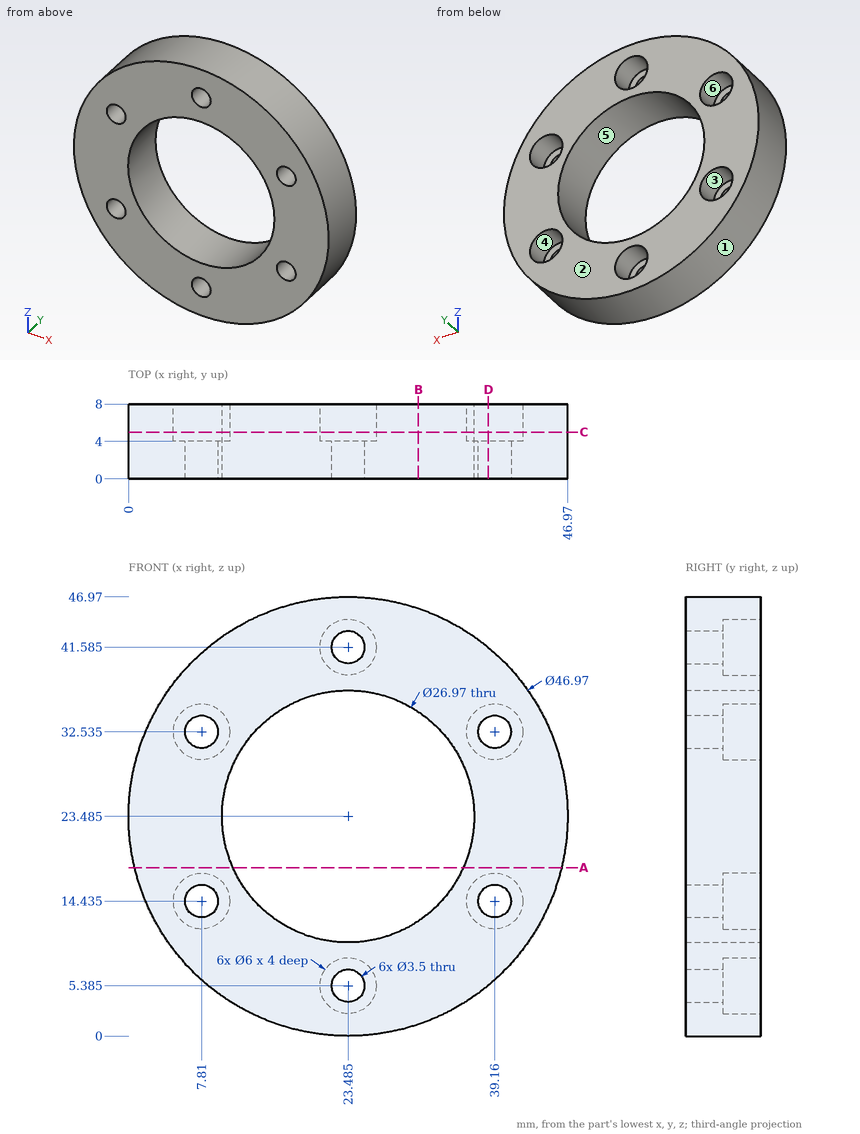
Can you work these out from the drawing? Everything is in mm from the part's minimum corner. A direction names the side the tool comes from. Round coordinates to 2 decimals unless told otherwise and drop trailing zeros. Loops run counter-clockwise (first coordinate to the right, second up) from the corner with the lowest first, then second, coordinate; pieces in that order, holes last. Notation, with made-up numbers: (-18, -29.75) - (-8, -29.75) arc R15 ccw to (-8, -17.75) - close; hole circle Ø4 at (-8.5, -23). An arc over 180 degrees is marked (long way). One line per question, with ' | ' between items. Start each with the question number.
Q1. We'd pull the mould along Z, two halves only. Please class the marked faces 1, 2, 3 and 4: +Z half, -Z half, draft (parallel to the pull), parting line (faces both ways), or undercut.
Q2. I want a section at A-A (z = 18). Write out the boundary of the cut face in (x, y).
Q3. I want a section at B-B (x = 31). Write out the boundary of the cut face in (y, z).
Q4. I want a section at D-D (x = 38.5). Write out the boundary of the cut face in (y, z), then the cut area to 3 significant figures.
Q5. I want a section at C-C (y = 5). Write out the boundary of the cut face in (x, z) (3 decimals).
Q6. Please list where these lines run through material, in increasing order: line 1 (X direction, y = 3, z = 14) (1 decimal); line 2 (X direction, y = 6.25, z = 34); line 3 (Z direction, x = 23, y = 6.75) (1 decimal). Write a range as [from, to].
Q7. Will these pins go through, and if not, where does the flat tip stop? pin 1 (4 mm diameter, centred on x = 23.485, z = 41.585, fed in from -Y); pin 2 (1.8 mm diameter, centred on x = 7, z = 13.5, fed in from +Y); pin 3 (3 mm diameter, centred on x = 7.81, z = 32.53, fed in from -Y); pin 4 (4 mm diameter, centred on x = 33, y = 6, fed in from -Z).
Q8. For the marked faces 5 and 6, which set-ups out of +Z, -Z, +X, -X, +Y, -Y let a thin tool reach every point of the face, with its end or its side?
Response values:
1) face 1: parting line | face 2: draft | face 3: undercut | face 4: undercut
2) outline: (0.65, 0) - (11.17, 0) - (11.17, 8) - (0.65, 8) - close; (35.8, 0) - (46.32, 0) - (46.32, 8) - (35.8, 8) - close
3) outline: (0, 1.23) - (8, 1.23) - (8, 12.29) - (0, 12.29) - close; (0, 34.68) - (8, 34.68) - (8, 45.74) - (0, 45.74) - close
4) outline: (0, 5.43) - (8, 5.43) - (8, 11.51) - (4, 11.51) - (4, 12.81) - (0, 12.81) - close; (0, 16.06) - (4, 16.06) - (4, 17.36) - (8, 17.36) - (8, 29.61) - (4, 29.61) - (4, 30.91) - (0, 30.91) - close; (0, 34.16) - (4, 34.16) - (4, 35.46) - (8, 35.46) - (8, 41.54) - (0, 41.54) - close | area: 216 mm²
5) outline: circle Ø46.97 at (23.485, 23.485); hole circle Ø6 at (7.81, 14.435); hole circle Ø6 at (7.81, 32.535); hole circle Ø26.97 at (23.485, 23.485); hole circle Ø6 at (23.485, 5.385); hole circle Ø6 at (23.485, 41.585); hole circle Ø6 at (39.16, 14.435); hole circle Ø6 at (39.16, 32.535)
6) line 1: x = [2, 6.1], [9.5, 13.9], [33.1, 37.5], [40.9, 45] | line 2: x = [2.49, 5.19], [10.43, 15.04], [31.93, 36.54], [41.78, 44.48] | line 3: z = [0, 2.4], [8.3, 10], [37, 38.6], [44.5, 47]
7) pin 1: stops at y = 0 | pin 2: stops at y = 4 | pin 3: passes through | pin 4: stops at z = 1.23
8) face 5: +Y, -Y | face 6: +Y
